The listing builds one solid part. Answer for the finished solid, in the listing's coordinates (mm). A direction names the side the tool comes from. Round coordinates to 2 decimals unless told otherwise and drop trailing zeros. Write each loop counter-clockwise with the first axis right and the second up, starting at its lowest first coordinate (ties: lowest second). Pieces come first, ordered by that corner, then holes. Notation, with made-up numbers: (43, 37.25) - (56, 37.25) arc R13 ccw to (56, 47.25) - close; hole circle Ø1 at (21, 61). An arc over 180 degrees is marked (long way). Answer as CSV lines item,"result". Start each with the question number.
Item 1: A cutting plane is placed at C-C on y = 18. Determine the outline of the cut face in (x, z) (3 decimals).
Item 2: A cutting plane is placed at B-B on z = 4. Determine the outline of the cut face in (x, y) (3 decimals).
Item 3: For a pull along X with two mould halves and no side action, classify faces 1 (the flat face through (-15.24, 33, 20)), 2 (the cylindrical face through (1.29, 2.024, 36.159)), 3 (the flat face through (-16, 13, 33.655)), 4 (the cylindrical face through (6.83, -6.64, 2.5)) as pulls with the +X half, pulls with the -X half, needs draft (parallel to the pull), parting line crosses it, or undercut.
Item 4: Straight lines are drawn through the part: line 1 along Z through (x, y) = (-35, 23) (3 decimals); line 2 along Y through (x, z) = (0, 37.15) (3 decimals); line 3 along Y through (x, z) = (-31.5, 19). For each, find the intervals that lie inside material, in ascending order. Write a range as [from, to].
Item 5: A cutting plane is placed at A-A on x = -27.94. Determine the outline of the cut face in (y, z) (1 decimal).
Item 6: Which of the six approach directions +Z, -Z, +X, -X, +Y, -Y give full straight-line access (tool end or side, diameter ignored) to faces 5 (the flat face through (-16, 13, 0)), 6 (the flat face through (-31, 31.877, 20))?
Item 7: A cutting plane is placed at D-D on x = 0. Determine the outline of the cut face in (y, z) (3 decimals), and give its area (3 significant figures).
Item 8: Flat-ended cylindrical pins translate along their axes: pin 1 (3.5 mm diameter, centred on y = 33, z = 22.5, fed in from +X); pin 2 (12 mm diameter, centred on y = 18, z = 33, fed in from +X); pin 3 (5 mm diameter, centred on x = -21.5, z = 24.5, fed in from -Y). Find the tip coordinate at first contact, or state that the pin passes through.
```python
from build123d import *

# Parameters (mm, degrees)
SKETCH1_W            = 25.4
SKETCH1_H            = 19.05
SKETCH1_R            = 9.525
BOSS_EXTRUDE1_DEPTH  = 5.08
M4_CLEARANCE_HOLE1_D = 4.8
SKETCH4_W            = 25.4
SKETCH4_H            = 3.175
BOSS_EXTRUDE2_DEPTH  = 14.2875
M5_CLEARANCE_HOLE1_D = 5.8
FILLET1_R            = 6.35


with BuildPart() as part:
    # Sketch1 → Boss-Extrude1 (new body)
    with BuildSketch(Plane.XY):
        with Locations((-27.94, 25.527)):
            Rectangle(SKETCH1_W, SKETCH1_H)
        with BuildLine():
            Line((-15.24, 16.002), (-40.64, 16.002))
            Line((-40.64, 16.002), (-5.338467717, -7.888370392))
            ThreePointArc((-5.338467717, -7.888370392), (-6.957108321, 6.505710477), (7.51306662, 5.854865922))
            Line((7.51306662, 5.854865922), (-15.24, 35.052))
            Line((-15.24, 35.052), (-15.24, 16.002))
        make_face()
        Circle(SKETCH1_R)
    extrude(amount=BOSS_EXTRUDE1_DEPTH)

    # M4 Clearance Hole1 (through all)
    with Locations(Plane(origin=(0, 0, 0), x_dir=(-1, 0, 0), z_dir=(0, 0, -1))):
        with Locations((0, 0)):
            Hole(M4_CLEARANCE_HOLE1_D / 2)

    # Sketch4 → Boss-Extrude2 (add)
    with BuildSketch(Plane.XY.offset(5.08)):
        with Locations((-27.94, 33.4645)):
            Rectangle(SKETCH4_W, SKETCH4_H)
    extrude(amount=BOSS_EXTRUDE2_DEPTH)

    # Mirror3: part across plane


with BuildPart() as part_1:
    add(part.part)
    add(part.part.mirror(Plane.XY.offset(19.3675)))

    # M5 Clearance Hole1 (through all)
    with Locations(Plane(origin=(0, 35.052, 0), x_dir=(1, 0, 0), z_dir=(0, 1, 0))):
        with Locations((-27.94, -19.3675)):
            Hole(M5_CLEARANCE_HOLE1_D / 2)

    # Fillet1
    fillet1_edges = [part_1.edges().sort_by_distance(p)[0] for p in [
        (-40.64, 16.002, 2.54),
        (-40.64, 16.002, 36.195),
    ]]
    fillet(fillet1_edges, radius=FILLET1_R)


solid = part_1.part
```
Geometry says:
1,outline,"(-40.49, 0) - (-1.952, 0) - (-1.952, 5.08) - (-40.49, 5.08) - close; (-40.49, 33.655) - (-1.952, 33.655) - (-1.952, 38.735) - (-40.49, 38.735) - close"
2,outline,"(-40.64, 19.372) arc R6.35 ccw to (-37.849, 14.113) - (-5.338, -7.888) arc R9.525 ccw to (7.513, 5.855) - (-15.24, 35.052) - (-40.64, 35.052) - close; hole circle Ø4.8 at (0, 0)"
3,face 1,"pulls with the +X half"
3,face 2,"undercut"
3,face 3,"needs draft"
3,face 4,"parting line crosses it"
4,line 1,"z = [0, 5.08], [33.655, 38.735]"
4,line 2,"y = [-9.525, -2.4], [2.4, 15.496]"
4,line 3,"y = [31.88, 35.05]"
5,outline,"(7.4, 0) - (35.1, 0) - (35.1, 16.5) - (31.9, 16.5) - (31.9, 5.1) - (7.4, 5.1) - close; (7.4, 33.7) - (31.9, 33.7) - (31.9, 22.3) - (35.1, 22.3) - (35.1, 38.7) - (7.4, 38.7) - close"
6,face 5,"-Z, +X, -X, +Y, -Y"
6,face 6,"+X, -X, -Y"
7,outline,"(-9.525, 0) - (-2.4, 0) - (-2.4, 5.08) - (-9.525, 5.08) - close; (-9.525, 33.655) - (-2.4, 33.655) - (-2.4, 38.735) - (-9.525, 38.735) - close; (2.4, 0) - (15.496, 0) - (15.496, 5.08) - (2.4, 5.08) - close; (2.4, 33.655) - (15.496, 33.655) - (15.496, 38.735) - (2.4, 38.735) - close"
7,area,"205 mm^2"
8,pin 1,"stops at x = -15.24"
8,pin 2,"stops at x = 2.7"
8,pin 3,"stops at y = 31.88"
